from build123d import *

# Parameters (mm, degrees)
F0_R     = 1.6
F1_DEPTH = 3.175


with BuildPart() as f1:
    # F0 (on Top) → F1 (new body)
    with BuildSketch(Plane.XY):
        with BuildLine():
            ThreePointArc((0, -6.35), (7.207455, 0), (0, 6.35))
            Line((0, 6.35), (-30, 2.54))
            ThreePointArc((-30, 2.54), (-32.237822, 0), (-30, -2.54))
            Line((-30, -2.54), (0, -6.35))
        make_face()
        with Locations((-29.271, 0)):
            Circle(F0_R, mode=Mode.SUBTRACT)
        with Locations((-19.271, 0)):
            Circle(F0_R, mode=Mode.SUBTRACT)
        with Locations((-9.271, 0)):
            Circle(F0_R, mode=Mode.SUBTRACT)
        Polygon((-2.313127, 1.150841), (-2.481189, 1.651718), (-1.954254, 1.689937), (-1.992473, 2.216873), (-1.472587, 2.122848), (-1.378562, 2.642733), (-0.898392, 2.422372), (-0.678031, 2.902541), (-0.267748, 2.56969), (0.065104, 2.979972), (0.37972, 2.555544), (0.804147, 2.87016), (1.003328, 2.380825), (1.492663, 2.580005), (1.563894, 2.056509), (2.08739, 2.12774), (2.026194, 1.602976), (2.550958, 1.54178), (2.361181, 1.048721), (2.85424, 0.858945), (2.547807, 0.428572), (2.97818, 0.122139), (2.574344, -0.218506), (2.914989, -0.622342), (2.439126, -0.851855), (2.668639, -1.327718), (2.150649, -1.431678), (2.254609, -1.949669), (1.727038, -1.921544), (1.698914, -2.449115), (1.194912, -2.290672), (1.036469, -2.794674), (0.587704, -2.515869), (0.308899, -2.964634), (-0.056431, -2.582985), (-0.43808, -2.948314), (-0.69702, -2.487802), (-1.157533, -2.746742), (-1.293813, -2.236301), (-1.804254, -2.372581), (-1.809311, -1.844285), (-2.337607, -1.849342), (-2.211123, -1.336386), (-2.724079, -1.209903), (-2.474002, -0.744517), (-2.939388, -0.494441), (-2.581431, -0.105868), (-2.970004, 0.252089), (-2.526659, 0.539434), (-2.814004, 0.982779), align=None, mode=Mode.SUBTRACT)
    extrude(amount=F1_DEPTH)


solid = f1.part
Can you work these out from the model? Positions are in its coordinate system, mm. Round coordinates to 2 decimals unless told otherwise and drop trailing zeros. Loops run counter-clockwise (first coordinate to the right, second up) from the corner with the lowest first, then second, coordinate; pieces in that order, holes last. Notation, with made-up numbers: (29, 27) - (47, 27) arc R4 ccw to (47, 33) - close; hole circle Ø9 at (37.25, 60). An arc over 180 degrees is marked (long way). Use CSV: the item, a comma, the result in double quotes. Start each with the question number.
1) If we section it at B-B on z = 0.6: Count the separate pieces of the cut face and the enclosed holes in it, plus the area to 3 significant figures.
2) We'd pull the mould along Y, two halves only. Please class faces 1 (the cylindrical face through (-7.79, -0.61, 1.57)), 2 (the cylindrical face through (-20.45, 1.08, 1.57)), 3 (the cylindrical face through (7.206, -0.152, 1.565)), 4 (the flat face through (-8, 2, 3.175)): released by +Y, released by -Y, zero draft, split by the parting line, or undercut.
3) If we section it at C-C on y = 4.5: Write out the boundary of the cut face in (x, z) (3 decimals).
4) Please list where these lines run through material, in increasing order: probe 1 along Y at (x, z) = (-0.5, 2.8); probe 2 along Y at (x, z) = (-28, 0.1); probe 3 along X at (y, z) = (-1.75, 1). Write a range as [from, to].
5) For pin 1 Ø1.5 at (x, z) = (-14, 1) entering from -Y, with a flat end and sliding along its axis, tell me the tip position at first contact or that it passes through.
6) If we section it at A-A on x = -20.5: Write out the boundary of the cut face in (y, z) (1 decimal).
7) If we section it at D-D on x = -4.5: Write out the boundary of the cut face in (y, z) (1 decimal).
Geometry results:
1,separate pieces,"1"
1,enclosed holes,"4"
1,area,"302 mm2"
2,face 1,"undercut"
2,face 2,"undercut"
2,face 3,"split by the parting line"
2,face 4,"zero draft"
3,outline,"(-14.567, 0) - (5.359, 0) - (5.359, 3.175) - (-14.567, 3.175) - close"
4,probe 1,"y = [-6.29, -2.84], [2.76, 6.29]"
4,probe 2,"y = [-2.79, -0.97], [0.97, 2.79]"
4,probe 3,"x = [-31.55, -2.31], [2.21, 6.96]"
5,pin 1,"stops at y = -4.67"
6,outline,"(-3.7, 0) - (-1, 0) - (-1, 3.2) - (-3.7, 3.2) - close; (1, 0) - (3.7, 0) - (3.7, 3.2) - (1, 3.2) - close"
7,outline,"(-5.8, 0) - (5.8, 0) - (5.8, 3.2) - (-5.8, 3.2) - close"
